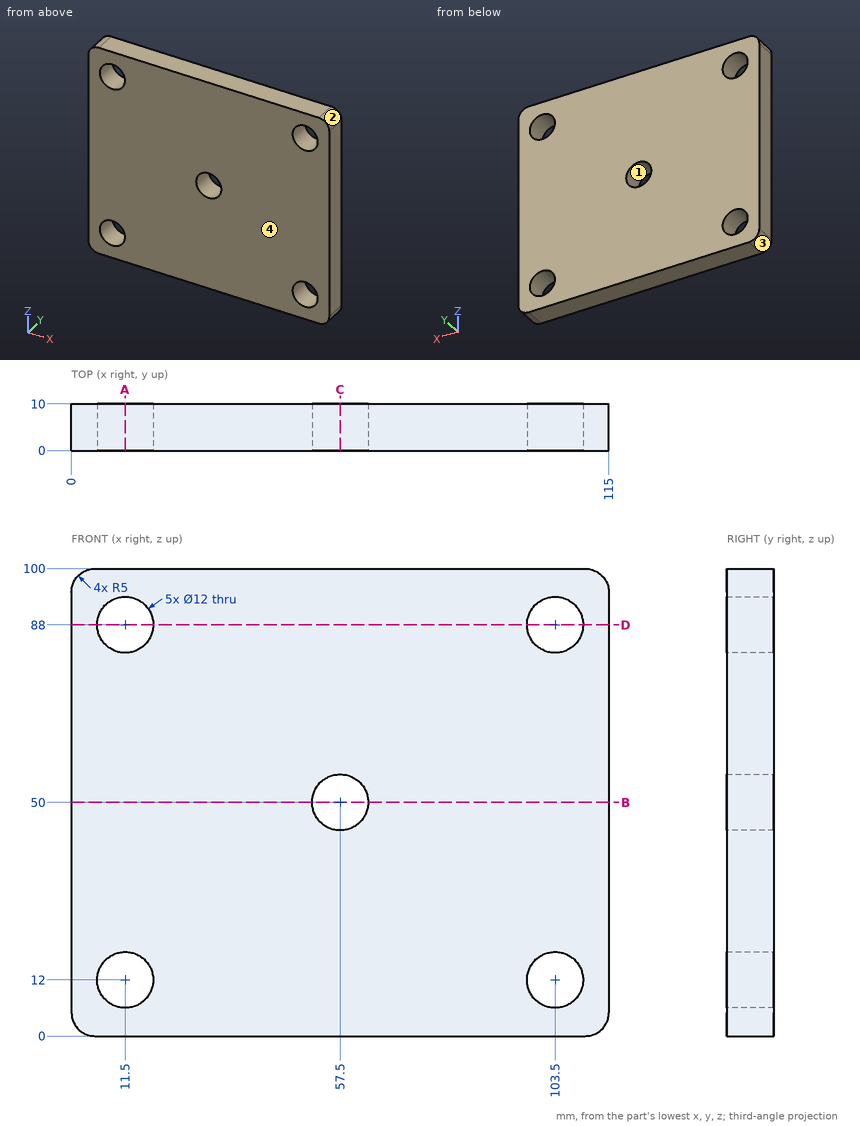
Answer from the drawing. Dimensions are ordinates in mm from the lowest x, y and z of the part. Round coordinates to 2 decimals unless told otherwise and drop trailing zeros. Write each loop counter-clockwise with the first axis right and the second up, starting at its lowest first coordinate (ties: lowest second). Pieces come first, ordered by that corner, then holes.
1. Given pin 1 Ø9.5 at (x, z) = (103.5, 12) entering from -Y, flat-ended and moving along its own axis, determine where the tip first touches the part or whether it passes through.
2. The part is cut by section B-B, the plane z = 50. Determine the outline of the cut face in (x, y), then the cut area to 3 significant figures.
3. Determine the mould class of the marked faces 1, 2, 3 and 4 for opening direction X: pulls with the +X half, pulls with the -X half, needs draft (parallel to the pull), parting line crosses it, or undercut.
4. The part is cut by section C-C, the plane x = 57.5. Determine the outline of the cut face in (y, z), then the cut area to 3 significant figures.
5. Straight lines are drawn through the part: L1, parallel to X at y = 5.75, z = 12; L2, parallel to Z at x = 58, y = 8; L3, parallel to X at y = 5.75, z = 50. For each, find the intervals that lie inside material, in ascending order.
6. The part is cut by section A-A, the plane x = 11.5. Determine the outline of the cut face in (y, z), then the cut area to 3 significant figures.
7. The part is cut by section D-D, the plane z = 88. Determine the outline of the cut face in (x, y).
Values:
1. pin 1: passes through
2. outline: (0, 0) - (51.5, 0) - (51.5, 10) - (0, 10) - close; (63.5, 0) - (115, 0) - (115, 10) - (63.5, 10) - close
2. area: 1,030 mm2
3. face 1: undercut
3. face 2: pulls with the +X half
3. face 3: pulls with the -X half
3. face 4: needs draft
4. outline: (0, 0) - (10, 0) - (10, 44) - (0, 44) - close; (0, 56) - (10, 56) - (10, 100) - (0, 100) - close
4. area: 880 mm2
5. L1: x = 0 to 5.5, 17.5 to 97.5, 109.5 to 115
5. L2: z = 0 to 44.02, 55.98 to 100
5. L3: x = 0 to 51.5, 63.5 to 115
6. outline: (0, 0) - (10, 0) - (10, 6) - (0, 6) - close; (0, 18) - (10, 18) - (10, 82) - (0, 82) - close; (0, 94) - (10, 94) - (10, 100) - (0, 100) - close
6. area: 760 mm2
7. outline: (0, 0) - (5.5, 0) - (5.5, 10) - (0, 10) - close; (17.5, 0) - (97.5, 0) - (97.5, 10) - (17.5, 10) - close; (109.5, 0) - (115, 0) - (115, 10) - (109.5, 10) - close
